Could you check a few things on this model? Use its own coordinates, in mm. A direction names the side the tool comes from. Round coordinates to 2 decimals unless told otherwise and drop trailing zeros. Loops run counter-clockwise (first coordinate to the right, second up) from the corner with the lowest first, then second, coordinate; pieces in that order, holes last. Notation, with made-up numbers: M 19.25,68 L 41.25,68 A25 cw 41.25,104 Z; hole C 62.5,-7.5 d9. An arc over 180 degrees is marked long. One line per item, written item: value. Start each with the question number.
Q1. Please list where these lines run through material, in increasing order: line 1 along Y through (x, z) = (31, 0.1); line 2 along Z through (x, y) = (14, 1.5); line 3 along Y through (x, z) = (8.5, 0.25).
Q2. I'm going to push flat-ended pins straight in: pin 1 Ø2.5 at (x, y) = (31, 0) entering from -Z; pin 2 Ø1.5 at (x, z) = (4.5, -2.5) entering from -Y; pin 3 Ø2 at (x, z) = (21, -2) entering from -Y. Where does each tip first touch, or does it pass through?
Q3. Imagine slicing it at C-C (x = 7). Please give me the cut outline in (y, z).
Q4. Imagine slicing it at B-B (z = 0). Please give me the cut outline in (x, y).
Q5. Which directions (+Z, -Z, +X, -X, +Y, -Y) give clear straight access to the entire face, cutting with the end or side of a thin tool? Please do faces 1 (the face through (29, 0, -1.5)), 2 (the face through (29, 0, 1.5)).
Q6. Thinking about a two-plate mould opening in Y: for faces 3 (the face through (16, 0, -4)), 4 (the face through (30, 0, 0)), 5 (the face through (0, 0, 0)), which applies, released by +Y, released by -Y, zero draft, split by the parting line, or undercut?
Q7. Imagine slicing it at A-A (y = 0). Please give me the cut outline in (x, z).
from build123d import *

# Parameters (mm, degrees)
F2_SIZE  = 0.5
F4_START = -1.5
F4_DEPTH = 6.5
F5_R     = 1
F6_DEPTH = 1.5


# Not quite as in the source:
# - a pattern or mirror of a feature is missing from the dataset's text; its kind, count and spacing are read off the source's solid


with BuildPart() as f1:
    # F0 (on Front) → F1 (revolve)
    with BuildSketch(Plane.XZ):
        with BuildLine():
            Line((0, 4), (0, 0))
            Line((0, 0), (35, 0))
            ThreePointArc((35, 0), (33.8284271247, 2.8284271247), (31, 4))
            Line((31, 4), (0, 4))
        make_face()
    revolve(axis=Axis((22.9748431593, 0, 0), (1, 0, 0)))

    # F2
    f2_edges = [f1.edges().sort_by_distance(p)[0] for p in [
        (0, 0, -4),
    ]]
    chamfer(f2_edges, length=F2_SIZE)

    # F3 (on Top) → F4 (cut)
    with BuildSketch(Plane.XY.offset(F4_START)):
        with BuildLine():
            Line((26, -4), (31, -4))
            ThreePointArc((31, -4), (35, 0), (31, 4))
            Line((31, 4), (26, 4))
            Line((26, 4), (26, -4))
        make_face()
    f4 = extrude(amount=-F4_DEPTH, mode=Mode.SUBTRACT)

    # F4_copies: F4 across plane
    add(f4.mirror(Plane.XY), mode=Mode.SUBTRACT)

    # F5 (on Top) → F6 (cut, symmetric)
    with BuildSketch(Plane.XY):
        with Locations((31, 0)):
            Circle(F5_R)
    extrude(amount=F6_DEPTH, both=True, mode=Mode.SUBTRACT)


solid = f1.part
Report:
1. line 1: y = -4 to -1, 1 to 4
1. line 2: z = -3.71 to 3.71
1. line 3: y = -3.99 to 3.99
2. pin 1: stops at z = -1.5
2. pin 2: stops at y = -3.6
2. pin 3: stops at y = -3.87
3. outline: C 0,0 d8
4. outline: M 0,-3.5 L 0.5,-4 L 31,-4 A4 ccw 31,4 L 0.5,4 L 0,3.5 Z; hole C 31,0 d2
5. face 1: -Z, +X, +Y, -Y
5. face 2: +Z, +X, +Y, -Y
6. face 3: split by the parting line
6. face 4: undercut
6. face 5: zero draft
7. outline: M 0,-3.5 L 0.5,-4 L 26,-4 L 26,-1.5 L 30,-1.5 L 30,1.5 L 26,1.5 L 26,4 L 0.5,4 L 0,3.5 Z; M 32,-1.5 L 34.71,-1.5 A4 ccw 34.71,1.5 L 32,1.5 Z
